Read the model definition and answer for the solid it produces. Units are mm, in the model's axes. Round coordinates to 2 decimals unless told otherwise and drop trailing zeros. Order: outer loops, then holes, each group sorted by start corner. A loop starts at its lowest first (then second) coordinate and runs counter-clockwise, first axis right, second up. Notation, with made-up numbers: (-3.75, -19.5) - (31.25, -19.5) arc R12 ccw to (31.25, 2.5) - close; hole circle Ø3 at (8.25, 74). An arc over 180 degrees is marked (long way). Answer as a JSON object with one key per item and string values. Group by question number.
Q1. A cutting plane is placed at D-D on x = 48. Determine the outline of the cut face in (y, z).
Q2. A cutting plane is placed at B-B on z = -2. Determine the outline of the cut face in (x, y), and give its area (3 significant figures).
Q3. A cutting plane is placed at A-A on x = 33. Determine the outline of the cut face in (y, z), and give its area (3 significant figures).
Q4. Given pin 1 Ø1.2 at (y, z) = (2, 6.5) entering from -X; pin 2 Ø5 at (x, z) = (33.5, 18) entering from -Y; pin 3 Ø2 at (x, y) = (115.5, 1.5) entering from -Z; pin 4 Ø2 at (y, z) = (1.5, 6.5) entering from +X, each flat-ended and moving along its own axis, determine where each tip first touches the part or whether it passes through.
Q5. Consider line 1 (X direction, y = 1.4, z = -2.5); line 2 (X direction, y = 1.55, z = 5.5); line 3 (Z direction, x = 115.5, y = 2.05). Determine where each line is inside the solid, lowest interval first.
Q6. A cutting plane is placed at C-C on y = 1.7. Count the separate pieces of the cut face and the enclosed holes in it, and give its area (3 significant figures).
```python
from build123d import *

# Parameters (mm, degrees)
SKETCH1_W           = 121
SKETCH1_H           = 25
BOSS_EXTRUDE1_DEPTH = 4
SKETCH2_W           = 4
SKETCH2_H           = 5
BOSS_EXTRUDE2_DEPTH = 4
LPATTERN1_COUNT     = 3
LPATTERN1_PITCH     = 10
SKETCH3_W           = 10
SKETCH3_H           = 4
BOSS_EXTRUDE3_DEPTH = 4
LPATTERN2_COUNT     = 3
LPATTERN2_PITCH     = 20
LPATTERN2_COL_COUNT = 3
LPATTERN2_COL_PITCH = 20
SKETCH4_W           = 10
SKETCH4_H           = 4
CUT_EXTRUDE1_DEPTH  = 128.538229563
SKETCH5_R           = 1.5
SKETCH5_W           = 12
SKETCH5_H           = 9
CUT_EXTRUDE2_DEPTH  = 128.538229563
SKETCH7_W           = 4
SKETCH7_H           = 4
CUT_EXTRUDE4_DEPTH  = 128.538229563


with BuildPart() as part:
    # Sketch1 → Boss-Extrude1 (new body)
    with BuildSketch(Plane(origin=(0, 0, 0), x_dir=(1, 0, 0), z_dir=(0, 1, 0))):
        with Locations((60.5, -12.5)):
            Rectangle(SKETCH1_W, SKETCH1_H)
    extrude(amount=BOSS_EXTRUDE1_DEPTH)

    # Sketch2 → Boss-Extrude2 (add, through all)
    with BuildSketch(Plane(origin=(0, 0, 0), x_dir=(-1, 0, 0), z_dir=(0, -1, 0))):
        with Locations((2, -22.5)):
            Rectangle(SKETCH2_W, SKETCH2_H)
        with Locations((-123, -22.5)):
            Rectangle(SKETCH2_W, SKETCH2_H)
    boss_extrude2 = extrude(amount=-BOSS_EXTRUDE2_DEPTH)

    # LPattern1: Boss-Extrude2 ×3
    with Locations(*[(0, 0, -i * LPATTERN1_PITCH) for i in range(1, LPATTERN1_COUNT)]):
        add(boss_extrude2)

    # Sketch3 → Boss-Extrude3 (add, through all)
    with BuildSketch(Plane(origin=(0, 0, 0), x_dir=(-1, 0, 0), z_dir=(0, -1, 0))):
        with Locations((-60.5, 2)):
            Rectangle(SKETCH3_W, SKETCH3_H)
    boss_extrude3 = extrude(amount=-BOSS_EXTRUDE3_DEPTH)

    # LPattern2: Boss-Extrude3 ×3
    with Locations(*[(i * LPATTERN2_PITCH, 0, 0) for i in range(1, LPATTERN2_COUNT)]):
        add(boss_extrude3)

    # LPattern2 col: Boss-Extrude3 ×3
    with Locations(*[(-i * LPATTERN2_COL_PITCH, 0, 0) for i in range(1, LPATTERN2_COL_COUNT)]):
        add(boss_extrude3)

    # Sketch4 → Cut-Extrude1 (cut, through all)
    with BuildSketch(Plane.XZ):
        with Locations((20.5, 6)):
            Rectangle(SKETCH4_W, SKETCH4_H)
        with Locations((40.5, 6)):
            Rectangle(SKETCH4_W, SKETCH4_H)
        with Locations((60.5, 6)):
            Rectangle(SKETCH4_W, SKETCH4_H)
        with Locations((80.5, 6)):
            Rectangle(SKETCH4_W, SKETCH4_H)
        with Locations((100.5, 6)):
            Rectangle(SKETCH4_W, SKETCH4_H)
    extrude(amount=-CUT_EXTRUDE1_DEPTH, mode=Mode.SUBTRACT)

    # Sketch5 → Cut-Extrude2 (cut, through all)
    with BuildSketch(Plane(origin=(0, 4, 0), x_dir=(1, 0, 0), z_dir=(0, 1, 0))):
        with Locations(Location((97.5, -13, 0), (0, 0, 270))):
            Circle(SKETCH5_R)
        with Locations(Location((102.5, -13, 0), (0, 0, 270))):
            Circle(SKETCH5_R)
        with Locations(Location((43, -13, 0), (0, 0, 270))):
            Circle(SKETCH5_R)
        with Locations(Location((38, -13, 0), (0, 0, 270))):
            Circle(SKETCH5_R)
        with Locations(Location((33, -13, 0), (0, 0, 270))):
            Circle(SKETCH5_R)
        with Locations(Location((28, -13, 0), (0, 0, 270))):
            Circle(SKETCH5_R)
        with Locations(Location((23, -13, 0), (0, 0, 270))):
            Circle(SKETCH5_R)
        with Locations(Location((18, -13, 0), (0, 0, 270))):
            Circle(SKETCH5_R)
        with Locations((60.5, -12.5)):
            Rectangle(SKETCH5_W, SKETCH5_H)
    extrude(amount=-CUT_EXTRUDE2_DEPTH, mode=Mode.SUBTRACT)

    # Sketch7 → Cut-Extrude4 (cut, through all)
    with BuildSketch(Plane.XZ):
        with Locations((6, 20)):
            Rectangle(SKETCH7_W, SKETCH7_H)
        with Locations((14, 20)):
            Rectangle(SKETCH7_W, SKETCH7_H)
        with Locations((6, 12)):
            Rectangle(SKETCH7_W, SKETCH7_H)
        with Locations((14, 12)):
            Rectangle(SKETCH7_W, SKETCH7_H)
        with Locations((107, 20)):
            Rectangle(SKETCH7_W, SKETCH7_H)
        with Locations((107, 12)):
            Rectangle(SKETCH7_W, SKETCH7_H)
        with Locations((115, 20)):
            Rectangle(SKETCH7_W, SKETCH7_H)
        with Locations((115, 12)):
            Rectangle(SKETCH7_W, SKETCH7_H)
    extrude(amount=-CUT_EXTRUDE4_DEPTH, mode=Mode.SUBTRACT)


solid = part.part
```
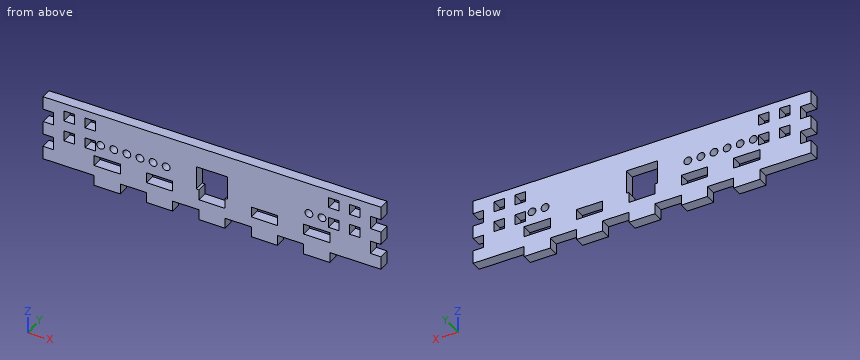
Result set:
{
 "1": {"outline": "(0, 0) - (4, 0) - (4, 25) - (0, 25) - close"},
 "2": {"outline": "(15.5, 0) - (25.5, 0) - (25.5, 4) - (15.5, 4) - close; (35.5, 0) - (45.5, 0) - (45.5, 4) - (35.5, 4) - close; (55.5, 0) - (65.5, 0) - (65.5, 4) - (55.5, 4) - close; (75.5, 0) - (85.5, 0) - (85.5, 4) - (75.5, 4) - close; (95.5, 0) - (105.5, 0) - (105.5, 4) - (95.5, 4) - close", "area": "200 mm²"},
 "3": {"outline": "(0, 0) - (4, 0) - (4, 11.5) - (0, 11.5) - close; (0, 14.5) - (4, 14.5) - (4, 25) - (0, 25) - close", "area": "88.0 mm²"},
 "4": {"pin 1": "stops at x = 0", "pin 2": "stops at y = 0", "pin 3": "stops at z = 0", "pin 4": "stops at x = 121"},
 "5": {"line 1": "x = 15.5 to 25.5, 35.5 to 45.5, 55.5 to 65.5, 75.5 to 85.5, 95.5 to 105.5", "line 2": "x = 0 to 15.5, 25.5 to 35.5, 45.5 to 55.5, 65.5 to 75.5, 85.5 to 95.5, 105.5 to 121", "line 3": "z = 0 to 10, 14 to 18, 22 to 25"},
 "6": {"separate pieces": "1", "enclosed holes": "21", "area": "2,850 mm²"}
}
